Geometry check sheet. Reference: the model listing, model coordinates, mm. A direction names the side the tool comes from. Round coordinates to 2 decimals unless told otherwise and drop trailing zeros. Write each loop counter-clockwise with the first axis right and the second up, starting at its lowest first coordinate (ties: lowest second). Pieces come first, ordered by that corner, then holes. Notation, with made-up numbers: (16.25, 53) -> (20.25, 53) arc R13 ccw to (20.25, 74) -> close; hole circle Ø7 at (23.5, -29). An arc over 180 degrees is marked (long way). Put each result on its own line as item: value. Start each with the question number.
from build123d import *
from build123d.topology import SkipClean

# Parameters (mm, degrees)
EXTRUDE_1_DEPTH          = 12
SKETCH_2_W               = 174
SKETCH_2_H               = 80
EXTRUDE_2_DEPTH          = 7
CUT_EXTRUDE_1_DEPTH      = 180.0296327
CUT_EXTRUDE_1_DEPTH_BACK = 180.0296327
SKETCH_5_R               = 14
EXTRUDE_5_DEPTH          = 12
CUT_EXTRUDE_2_DEPTH      = 181.23213316
CUT_EXTRUDE_2_DEPTH_BACK = 181.23213316
SKETCH_11_R              = 11
CUT_EXTRUDE_3_DEPTH      = 180.029667439
CUT_EXTRUDE_3_DEPTH_BACK = 180.029667439
CUT_EXTRUDE_4_DEPTH      = 180.029667439
CUT_EXTRUDE_4_DEPTH_BACK = 180.029667439
CUT_EXTRUDE_6_DEPTH      = 180.029667439
CUT_EXTRUDE_6_DEPTH_BACK = 180.029667439
EXTRUDE_6_DEPTH          = 3
CUT_EXTRUDE_7_DEPTH      = 180.029667439
CUT_EXTRUDE_7_DEPTH_BACK = 180.029667439
SKETCH_19_R              = 2.5
CUT_EXTRUDE_8_DEPTH      = 160.660954506
CUT_EXTRUDE_8_DEPTH_BACK = 160.660954506
SKETCH_20_R              = 2.5
CUT_EXTRUDE_9_DEPTH      = 180.029667439
CUT_EXTRUDE_9_DEPTH_BACK = 180.029667439
SKETCH_21_R              = 1.5
FILLET_1_R               = 3
FILLET_2_R               = 3
FILLET_3_R               = 3
FILLET_START             = -7
FILLET_4_DEPTH           = 14
FILLET_5_R               = 3
FILLET_6_R               = 3


with BuildPart() as part:
    # 草图1 → 凸台-拉伸1 (new, symmetric)
    with BuildSketch(Plane.XY):
        with BuildLine():
            Line((0, 31), (0, -31))
            ThreePointArc((0, -31), (31, 0), (0, 31))
        make_face()
    extrude(amount=EXTRUDE_1_DEPTH, both=True)

    # 草图2 → 凸台-拉伸2 (add, symmetric)
    with BuildSketch(Plane.XY):
        with Locations((87, 0.393184881)):
            Rectangle(SKETCH_2_W, SKETCH_2_H)
    extrude(amount=EXTRUDE_2_DEPTH, both=True)

    # 草图4 → 切除-拉伸1 (cut, two sides: drawn at the far end of the back side and taken through both)
    with BuildSketch(Plane.XY.offset(-CUT_EXTRUDE_1_DEPTH_BACK)):
        with BuildLine():
            Line((0, 26), (0, -26))
            ThreePointArc((0, -26), (26, 0), (0, 26))
        make_face()
    extrude(amount=CUT_EXTRUDE_1_DEPTH + CUT_EXTRUDE_1_DEPTH_BACK, mode=Mode.SUBTRACT)

    # 草图5 → 凸台-拉伸5 (add, symmetric)
    with BuildSketch(Plane.XY):
        with Locations((160.000035743, 0.361549397)):
            Circle(SKETCH_5_R)
    extrude(amount=EXTRUDE_5_DEPTH, both=True)

    # 草图11 → 切除-拉伸2 (cut, two sides: drawn at the far end of the back side and taken through both)
    with BuildSketch(Plane.XY.offset(12).offset(-CUT_EXTRUDE_2_DEPTH_BACK)):
        with Locations((160.000035743, 0.361549397)):
            Circle(SKETCH_11_R)
    extrude(amount=CUT_EXTRUDE_2_DEPTH + CUT_EXTRUDE_2_DEPTH_BACK, mode=Mode.SUBTRACT)

    # 草图12 → 切除-拉伸3 (cut, two sides: drawn at the far end of the back side and taken through both)
    with BuildSketch(Plane.XY.offset(-CUT_EXTRUDE_3_DEPTH_BACK)):
        with BuildLine():
            ThreePointArc((150.998055783, -10.360593896), (165.91494405, -12.327574282), (174.000035743, 0.361549397))
            Line((174.000035743, 0.361549397), (174, -39.606815119))
            Line((174, -39.606815119), (20, -39.606815119))
            Line((20, -39.606815119), (20, -27.606815119))
            Line((20, -27.606815119), (150.998055783, -10.360593896))
        make_face()
    extrude(amount=CUT_EXTRUDE_3_DEPTH + CUT_EXTRUDE_3_DEPTH_BACK, mode=Mode.SUBTRACT)

    # 草图13 → 切除-拉伸4 (cut, two sides: drawn at the far end of the back side and taken through both)
    with BuildSketch(Plane.XY.offset(-CUT_EXTRUDE_4_DEPTH_BACK)):
        with BuildLine():
            Line((20, 28.393184881), (151.063550898, 11.138341063))
            ThreePointArc((151.063550898, 11.138341063), (165.939252971, 13.039313345), (174, 0.393184881))
            Line((174, 0.393184881), (174, 40.393184881))
            Line((174, 40.393184881), (20, 40.393184881))
            Line((20, 40.393184881), (20, 28.393184881))
        make_face()
    extrude(amount=CUT_EXTRUDE_4_DEPTH + CUT_EXTRUDE_4_DEPTH_BACK, mode=Mode.SUBTRACT)

    # 草图14 → 切除-拉伸6 (cut, two sides: drawn at the far end of the back side and taken through both)
    with SkipClean():  # the faces are left unmerged after this step: merging them gives an invalid solid
        with BuildSketch(Plane.XY.offset(-CUT_EXTRUDE_6_DEPTH_BACK)):
            with BuildLine():
                Line((147.02443227, 5.618327355), (21.724512141, 22.114374787))
                ThreePointArc((21.724512141, 22.114374787), (30.993578045, 0.630967477), (22.606548392, -21.21188275))
                Line((22.606548392, -21.21188275), (147.000250841, -4.835141138))
                ThreePointArc((147.000250841, -4.835141138), (146.000073201, 0.393934732), (147.02443227, 5.618327355))
            make_face()
        extrude(amount=CUT_EXTRUDE_6_DEPTH + CUT_EXTRUDE_6_DEPTH_BACK, mode=Mode.SUBTRACT)
    add(part.part.scale(1), mode=Mode.REPLACE)  # the faces are merged on a copy

    # 草图17 → 凸台-拉伸6 (add, symmetric)
    with BuildSketch(Plane.XY):
        with BuildLine():
            ThreePointArc((22.606548392, -21.21188275), (30.993578045, 0.630967477), (21.724512141, 22.114374787))
            Line((21.724512141, 22.114374787), (147.02443227, 5.618327355))
            ThreePointArc((147.02443227, 5.618327355), (146.000073201, 0.393934732), (147.000250841, -4.835141138))
            Line((147.000250841, -4.835141138), (22.606548392, -21.21188275))
        make_face()
    extrude(amount=EXTRUDE_6_DEPTH, both=True)

    # 草图19 → 切除-拉伸7 (cut, two sides: drawn at the far end of the back side and taken through both)
    with BuildSketch(Plane(origin=(0, 0, 0), x_dir=(0, 0, -1), z_dir=(1, 0, 0)).offset(-CUT_EXTRUDE_7_DEPTH_BACK)):
        with Locations((0, 34)):
            Circle(SKETCH_19_R)
    extrude(amount=CUT_EXTRUDE_7_DEPTH + CUT_EXTRUDE_7_DEPTH_BACK, mode=Mode.SUBTRACT)

    # 草图20 → 切除-拉伸8 (cut, two sides: drawn at the far end of the back side and taken through both)
    with BuildSketch(Plane(origin=(20, 0, 0), x_dir=(0, 0, -1), z_dir=(1, 0, 0)).offset(-CUT_EXTRUDE_8_DEPTH_BACK)):
        with Locations((0, -34)):
            Circle(SKETCH_20_R)
    extrude(amount=CUT_EXTRUDE_8_DEPTH + CUT_EXTRUDE_8_DEPTH_BACK, mode=Mode.SUBTRACT)

    # 草图21 → 切除-拉伸9 (cut, two sides: drawn at the far end of the back side and taken through both)
    with BuildSketch(Plane(origin=(0, 0, 0), x_dir=(0, 0, -1), z_dir=(1, 0, 0)).offset(-CUT_EXTRUDE_9_DEPTH_BACK)):
        Circle(SKETCH_21_R)
    extrude(amount=CUT_EXTRUDE_9_DEPTH + CUT_EXTRUDE_9_DEPTH_BACK, mode=Mode.SUBTRACT)

    # 圆角1
    fillet_1_edges = [part.edges().sort_by_distance(p)[0] for p in [
        (10, -39.606815119, 7),
        (10, -39.606815119, -7),
        (10, 40.393184881, -7),
        (10, 40.393184881, 7),
    ]]
    fillet(fillet_1_edges, radius=FILLET_1_R)

    # 圆角2
    fillet_2_edges = [part.edges().sort_by_distance(p)[0] for p in [
        (31, 0, -12),
        (31, 0, 12),
    ]]
    fillet(fillet_2_edges, radius=FILLET_2_R)

    # 圆角3
    fillet_3_edges = [part.edges().sort_by_distance(p)[0] for p in [
        (22.606548392, -21.21188275, -5),
        (21.724512141, 22.114374787, -5),
        (21.724512141, 22.114374787, 5),
        (22.606548392, -21.21188275, 5),
    ]]
    fillet(fillet_3_edges, radius=FILLET_3_R)

    # 圆角4: read off the stored shape, not the designer's step
    # 圆角4 outline → 圆角4 (add)
    with SkipClean():  # the faces are left unmerged after this step: merging them gives an invalid solid
        with BuildSketch(Plane.XY.offset(FILLET_START)):
            with BuildLine():
                Line((147.02443227, 5.618327355), (143.612514441, 6.067514858))
                ThreePointArc((143.612514441, 6.067514858), (145.628554658, 4.882976839), (146.18195349, 2.611127766))
                ThreePointArc((146.18195349, 2.611127766), (146.519078394, 4.138292564), (147.02443227, 5.618327355))
            make_face()
            with BuildLine():
                ThreePointArc((147.000250841, -4.835141138), (146.503487598, -3.359094119), (146.173743348, -1.837004355))
                ThreePointArc((146.173743348, -1.837004355), (145.615277586, -4.102360388), (143.602544983, -5.2824576))
                Line((143.602544983, -5.2824576), (147.000250841, -4.835141138))
            make_face()
        extrude(amount=FILLET_4_DEPTH)

    # 圆角5
    fillet_5_edges = [part.edges().sort_by_distance(p)[0] for p in [
        (30.99663104, 0.457016597, 3),
        (86.372516009, 13.603303614, 3),
        (26.213672417, 19.781211811, 3),
        (26.760813079, -18.963065606, 3),
        (146.000059591, 0.387389859, 3),
        (86.629049021, -12.78316064, 3),
        (145.628554658, 4.882976839, 3),
        (145.615277586, -4.102360388, 3),
    ]]
    fillet(fillet_5_edges, radius=FILLET_5_R)

    # 圆角6
    fillet_6_edges = [part.edges().sort_by_distance(p)[0] for p in [
        (30.99663104, 0.457016597, -3),
        (86.372516009, 13.603303614, -3),
        (26.760813079, -18.963065606, -3),
        (26.213672417, 19.781211811, -3),
        (146.000059591, 0.387389859, -3),
        (86.629049021, -12.78316064, -3),
        (145.615277586, -4.102360388, -3),
        (145.628554658, 4.882976839, -3),
    ]]
    fillet(fillet_6_edges, radius=FILLET_6_R)


solid = part.part
(1) Mould release check, pull along Z, two halves, no side actions. Record for faces 4 (the cylindrical face through (9.86, 36.11, -1.34)), 5 (the cylindrical face through (26.24, 19.82, -6.49)), 6 (the cylindrical face through (10.14, -38.75, 6.1)): +Z half, -Z half, draft (parallel to the pull), parting line (faces both ways), or undercut.
(2) Sectioned sample at A-A (y = 34). Record the cut outline in (x, z).
(3) Go/stop test with flat-tipped pins: pin 1 Ø3.5 at (y, z) = (-32, 2.5) entering from +X; pin 2 Ø17.5 at (x, y) = (67.5, 7) entering from +Z; pin 3 Ø4 at (x, z) = (59.5, 5) entering from -Y. Record where each tip stops, or that it passes through.
(4) Material ranges on L1, parallel to Y at x = 7, z = 0; L2, parallel to Z at x = 14, y = 34; L3, parallel to X at y = 1.5, z = 8, recorded low to high. Write a range as from..to.
(5) Set-up check for faces 1 (the flat face through (20, 37, 0)), 2 (the cylindrical face through (26.787, -19.002, -6.493)), 3 (the flat face through (70, -20, 7)): record each of +Z, -Z, +X, -X, +Y, -Y from which the full face is reachable in a straight line by a thin tool's end or side.
Found:
1. face 4: undercut
1. face 5: draft
1. face 6: +Z half
2. outline: (0, -7) -> (20, -7) -> (20, -2.5) -> (0, -2.5) -> close; (0, 2.5) -> (20, 2.5) -> (20, 7) -> (0, 7) -> close
3. pin 1: x = 20
3. pin 2: z = 4.78
3. pin 3: y = -22.67
4. L1: -39.61..-36.5, -31.5..-25.04, 25.04..31.5, 36.5..40.39
4. L2: -7..-2.5, 2.5..7
4. L3: 25.96..30.96, 146.05..149.06, 170.94..173.95
5. face 1: +Z, -Z, +X, +Y
5. face 2: -Z
5. face 3: +Z, -Y
